Source: CAD feature listing. Evaluate the final solid. Frame: model axes, mm. Coordinates: 2 decimals unless noted, no trailing zeros.
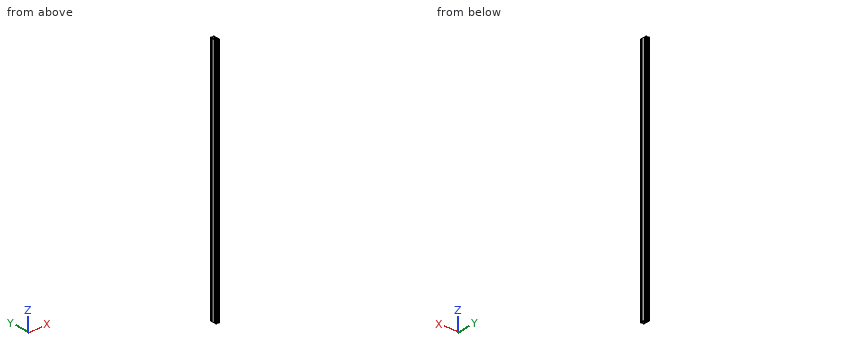
```python
from build123d import *

# Parameters (mm, degrees)
SKETCH1_R           = 3
SKETCH1_R_2         = 3.5
BOSS_EXTRUDE1_DEPTH = 2860


with BuildPart() as part:
    # Sketch1 → Boss-Extrude1 (new body)
    with BuildSketch(Plane.XY.offset(-2897)):
        with BuildLine():
            Line((-17, -40), (-4.1, -40))
            Line((-4.1, -40), (-4.1, -37))
            Line((-4.1, -37), (-10.5, -37))
            Line((-10.5, -37), (-10.5, -33.6627417))
            ThreePointArc((-10.5, -33.6627417), (-10.378207252, -33.050448208), (-10.03137085, -32.53137085))
            Line((-10.03137085, -32.53137085), (-7.464466094, -29.964466094))
            ThreePointArc((-7.464466094, -29.964466094), (-5.84234935, -28.880602337), (-3.928932188, -28.5))
            Line((-3.928932188, -28.5), (3.928932188, -28.5))
            ThreePointArc((3.928932188, -28.5), (5.84234935, -28.880602337), (7.464466094, -29.964466094))
            Line((7.464466094, -29.964466094), (10.03137085, -32.53137085))
            ThreePointArc((10.03137085, -32.53137085), (10.378207252, -33.050448208), (10.5, -33.6627417))
            Line((10.5, -33.6627417), (10.5, -37))
            Line((10.5, -37), (4.1, -37))
            Line((4.1, -37), (4.1, -40))
            Line((4.1, -40), (17, -40))
            ThreePointArc((17, -40), (19.121320344, -39.121320344), (20, -37))
            Line((20, -37), (20, -24.1))
            Line((20, -24.1), (17, -24.1))
            Line((17, -24.1), (17, -30.5))
            Line((17, -30.5), (13.6627417, -30.5))
            ThreePointArc((13.6627417, -30.5), (13.050448208, -30.378207252), (12.53137085, -30.03137085))
            Line((12.53137085, -30.03137085), (9.964466094, -27.464466094))
            ThreePointArc((9.964466094, -27.464466094), (8.880602337, -25.84234935), (8.5, -23.928932188))
            Line((8.5, -23.928932188), (8.5, -16.071067812))
            ThreePointArc((8.5, -16.071067812), (8.880602337, -14.15765065), (9.964466094, -12.535533906))
            Line((9.964466094, -12.535533906), (12.53137085, -9.96862915))
            ThreePointArc((12.53137085, -9.96862915), (13.050448208, -9.621792748), (13.6627417, -9.5))
            Line((13.6627417, -9.5), (17, -9.5))
            Line((17, -9.5), (17, -15.9))
            Line((17, -15.9), (20, -15.9))
            Line((20, -15.9), (20, 15.9))
            Line((20, 15.9), (17, 15.9))
            Line((17, 15.9), (17, 9.5))
            Line((17, 9.5), (13.6627417, 9.5))
            ThreePointArc((13.6627417, 9.5), (13.050448208, 9.621792748), (12.53137085, 9.96862915))
            Line((12.53137085, 9.96862915), (9.964466094, 12.535533906))
            ThreePointArc((9.964466094, 12.535533906), (8.880602337, 14.15765065), (8.5, 16.071067812))
            Line((8.5, 16.071067812), (8.5, 23.928932188))
            ThreePointArc((8.5, 23.928932188), (8.880602337, 25.84234935), (9.964466094, 27.464466094))
            Line((9.964466094, 27.464466094), (12.53137085, 30.03137085))
            ThreePointArc((12.53137085, 30.03137085), (13.050448208, 30.378207252), (13.6627417, 30.5))
            Line((13.6627417, 30.5), (17, 30.5))
            Line((17, 30.5), (17, 24.1))
            Line((17, 24.1), (20, 24.1))
            Line((20, 24.1), (20, 37))
            ThreePointArc((20, 37), (19.121320344, 39.121320344), (17, 40))
            Line((17, 40), (4.1, 40))
            Line((4.1, 40), (4.1, 37))
            Line((4.1, 37), (10.5, 37))
            Line((10.5, 37), (10.5, 33.6627417))
            ThreePointArc((10.5, 33.6627417), (10.378207252, 33.050448208), (10.03137085, 32.53137085))
            Line((10.03137085, 32.53137085), (7.464466094, 29.964466094))
            ThreePointArc((7.464466094, 29.964466094), (5.84234935, 28.880602337), (3.928932188, 28.5))
            Line((3.928932188, 28.5), (-3.928932188, 28.5))
            ThreePointArc((-3.928932188, 28.5), (-5.84234935, 28.880602337), (-7.464466094, 29.964466094))
            Line((-7.464466094, 29.964466094), (-10.03137085, 32.53137085))
            ThreePointArc((-10.03137085, 32.53137085), (-10.378207252, 33.050448208), (-10.5, 33.6627417))
            Line((-10.5, 33.6627417), (-10.5, 37))
            Line((-10.5, 37), (-4.1, 37))
            Line((-4.1, 37), (-4.1, 40))
            Line((-4.1, 40), (-17, 40))
            ThreePointArc((-17, 40), (-19.121320344, 39.121320344), (-20, 37))
            Line((-20, 37), (-20, 24.1))
            Line((-20, 24.1), (-17, 24.1))
            Line((-17, 24.1), (-17, 30.5))
            Line((-17, 30.5), (-13.6627417, 30.5))
            ThreePointArc((-13.6627417, 30.5), (-13.050448208, 30.378207252), (-12.53137085, 30.03137085))
            Line((-12.53137085, 30.03137085), (-9.964466094, 27.464466094))
            ThreePointArc((-9.964466094, 27.464466094), (-8.880602337, 25.84234935), (-8.5, 23.928932188))
            Line((-8.5, 23.928932188), (-8.5, 16.071067812))
            ThreePointArc((-8.5, 16.071067812), (-8.880602337, 14.15765065), (-9.964466094, 12.535533906))
            Line((-9.964466094, 12.535533906), (-12.53137085, 9.96862915))
            ThreePointArc((-12.53137085, 9.96862915), (-13.050448208, 9.621792748), (-13.6627417, 9.5))
            Line((-13.6627417, 9.5), (-17, 9.5))
            Line((-17, 9.5), (-17, 15.9))
            Line((-17, 15.9), (-20, 15.9))
            Line((-20, 15.9), (-20, -15.9))
            Line((-20, -15.9), (-17, -15.9))
            Line((-17, -15.9), (-17, -9.5))
            Line((-17, -9.5), (-13.6627417, -9.5))
            ThreePointArc((-13.6627417, -9.5), (-13.050448208, -9.621792748), (-12.53137085, -9.96862915))
            Line((-12.53137085, -9.96862915), (-9.964466094, -12.535533906))
            ThreePointArc((-9.964466094, -12.535533906), (-8.880602337, -14.15765065), (-8.5, -16.071067812))
            Line((-8.5, -16.071067812), (-8.5, -23.928932188))
            ThreePointArc((-8.5, -23.928932188), (-8.880602337, -25.84234935), (-9.964466094, -27.464466094))
            Line((-9.964466094, -27.464466094), (-12.53137085, -30.03137085))
            ThreePointArc((-12.53137085, -30.03137085), (-13.050448208, -30.378207252), (-13.6627417, -30.5))
            Line((-13.6627417, -30.5), (-17, -30.5))
            Line((-17, -30.5), (-17, -24.1))
            Line((-17, -24.1), (-20, -24.1))
            Line((-20, -24.1), (-20, -37))
            ThreePointArc((-20, -37), (-19.121320344, -39.121320344), (-17, -40))
        make_face()
        with Locations((15, 35)):
            Circle(SKETCH1_R, mode=Mode.SUBTRACT)
        with Locations((15, -35)):
            Circle(SKETCH1_R, mode=Mode.SUBTRACT)
        with Locations((0, 20)):
            Circle(SKETCH1_R_2, mode=Mode.SUBTRACT)
        with Locations((0, -20)):
            Circle(SKETCH1_R_2, mode=Mode.SUBTRACT)
        with Locations((-15, 35)):
            Circle(SKETCH1_R, mode=Mode.SUBTRACT)
        with Locations((-15, -35)):
            Circle(SKETCH1_R, mode=Mode.SUBTRACT)
        with BuildLine():
            Line((-14.242640687, -4.242640687), (-9.949747468, -8.535533906))
            ThreePointArc((-9.949747468, -8.535533906), (-8.327630724, -9.619397663), (-6.414213562, -10))
            Line((-6.414213562, -10), (6.414213562, -10))
            ThreePointArc((6.414213562, -10), (8.327630724, -9.619397663), (9.949747468, -8.535533906))
            Line((9.949747468, -8.535533906), (14.242640687, -4.242640687))
            ThreePointArc((14.242640687, -4.242640687), (16, 0), (14.242640687, 4.242640687))
            Line((14.242640687, 4.242640687), (9.949747468, 8.535533906))
            ThreePointArc((9.949747468, 8.535533906), (8.327630724, 9.619397663), (6.414213562, 10))
            Line((6.414213562, 10), (-6.414213562, 10))
            ThreePointArc((-6.414213562, 10), (-8.327630724, 9.619397663), (-9.949747468, 8.535533906))
            Line((-9.949747468, 8.535533906), (-14.242640687, 4.242640687))
            ThreePointArc((-14.242640687, 4.242640687), (-16, 0), (-14.242640687, -4.242640687))
        make_face(mode=Mode.SUBTRACT)
    extrude(amount=BOSS_EXTRUDE1_DEPTH)


solid = part.part
```
1. Section query A-A on z = -828. Count the separate pieces of the cut face and the enclosed holes in it, plus the area to 3 significant figures.
Findings:
separate pieces: 1
enclosed holes: 7
area: 1,390 mm2
2. Pin query (flat end, axial travel): P1, Ø0.9, axis at x = 18, z = -1614.5, coming from the -Y side; P2, Ø4, axis at y = -20.5, z = -1055.5, coming from the -X side; P3, Ø2.5, axis at x = -1.5, z = -1725, coming from the -Y side. Return the tip coordinate at first contact, or that it passes through.
Findings:
P1: stops at y = -39.95
P2: stops at x = -8.5
P3: stops at y = -28.5
3. Ray query, line 1 (Y direction, x = -15, z = -1027); line 2 (X direction, y = -11, z = -583); line 3 (Y direction, x = -1.5, z = -2530). Return the intervals inside material, ascending.
Findings:
line 1: y = -40 to -38, -32 to -30.5, -9.5 to -3.32, 3.32 to 9.5, 30.5 to 32, 38 to 40
line 2: x = -20 to -17, -11.5 to 11.5, 17 to 20
line 3: y = -28.5 to -23.16, -16.84 to -10, 10 to 16.84, 23.16 to 28.5
